Build history of the part. All positions in model axes, mm. A direction names the side the tool comes from. Coordinates: 2 decimals unless noted, no trailing zeros. Order: outer loops, then holes, each group sorted by start corner. A loop starts at its lowest first (then second) coordinate and runs counter-clockwise, first axis right, second up. Notation, with made-up numbers: (48.5, 39.5) - (71.5, 39.5) arc R29 ccw to (71.5, 78.5) - close; hole circle Ø11 at (-30.5, 44). An arc over 180 degrees is marked (long way). Return JSON: item names as keys, results as strings.
from build123d import *

# Parameters (mm, degrees)
SKIZZE1_W                       = 20
SKIZZE1_H                       = 18
SKIZZE1_R                       = 1.5
AUFSATZ_LINEAR_AUSTRAGEN1_DEPTH = 2
SKIZZE2_W                       = 0.8
SKIZZE2_H                       = 0.8
AUFSATZ_LINEAR_AUSTRAGEN2_DEPTH = 8
SKIZZE3_W                       = 1.5
SKIZZE3_H                       = 1.5
AUFSATZ_LINEAR_AUSTRAGEN3_DEPTH = 1.5
LINEARES_MUSTER1_COUNT          = 7
LINEARES_MUSTER1_PITCH          = 2.54


with BuildPart() as part:
    # Skizze1 → Aufsatz-Linear austragen1 (new body)
    with BuildSketch(Plane(origin=(0, 0, 0), x_dir=(1, 0, 0), z_dir=(0, 1, 0))):
        Rectangle(SKIZZE1_W, SKIZZE1_H)
        with Locations((-8, -7)):
            Circle(SKIZZE1_R, mode=Mode.SUBTRACT)
        with Locations((-8, 7)):
            Circle(SKIZZE1_R, mode=Mode.SUBTRACT)
    extrude(amount=AUFSATZ_LINEAR_AUSTRAGEN1_DEPTH)

    # Skizze2 → Aufsatz-Linear austragen2 (add)
    with BuildSketch(Plane.XZ):
        with Locations((8.6, 7.6)):
            Rectangle(SKIZZE2_W, SKIZZE2_H)
    aufsatz_linear_austragen2 = extrude(amount=AUFSATZ_LINEAR_AUSTRAGEN2_DEPTH)

    # Skizze3 → Aufsatz-Linear austragen3 (add)
    with BuildSketch(Plane(origin=(0, 0, 0), x_dir=(-1, 0, 0), z_dir=(0, -1, 0))):
        with Locations((-8.6, -7.6)):
            Rectangle(SKIZZE3_W, SKIZZE3_H)
    aufsatz_linear_austragen3 = extrude(amount=AUFSATZ_LINEAR_AUSTRAGEN3_DEPTH)

    # Lineares Muster1: Aufsatz-Linear austragen2, Aufsatz-Linear austragen3 ×7
    with Locations(*[(0, 0, -i * LINEARES_MUSTER1_PITCH) for i in range(1, LINEARES_MUSTER1_COUNT)]):
        add(aufsatz_linear_austragen2)
        add(aufsatz_linear_austragen3)


solid = part.part
1. Tool access for faces 4 (the flat face through (7.85, -1, 5)), 5 (the flat face through (9, -1, -8.39)), 6 (the flat face through (8.6, -8, 5.1)), 7 (the flat face through (8.6, -4.7, -0.42)), 8 (the flat face through (9, -5, -5)): list every direction of +Z, -Z, +X, -X, +Y, -Y with a clear straight run to the whole face (end or side of a thin tool).
Check values:
{"face 4": "+Z, -Z, -X, -Y", "face 5": "-Z, +X, -X, -Y", "face 6": "+Z, -Z, +X, -X, -Y", "face 7": "+X, -X, -Y", "face 8": "+Z, -Z, +X, -Y"}
2. Cut at A-A on x = -8. Give the cut face in (y, z), plus the area to 3 significant figures.
Check values:
{"outline": "(0, -9) - (2, -9) - (2, -8.5) - (0, -8.5) - close; (0, -5.5) - (2, -5.5) - (2, 5.5) - (0, 5.5) - close; (0, 8.5) - (2, 8.5) - (2, 9) - (0, 9) - close", "area": "24.0 mm²"}
3. Cut at B-B on z = 7.75. Give the cut face in (x, y).
Check values:
{"outline": "(-10, 0) - (-9.3, 0) - (-9.3, 2) - (-10, 2) - close; (-6.7, 0) - (7.85, 0) - (7.85, -1.5) - (8.2, -1.5) - (8.2, -8) - (9, -8) - (9, -1.5) - (9.35, -1.5) - (9.35, 0) - (10, 0) - (10, 2) - (-6.7, 2) - close"}
4. Probe L1, parallel to Z at x = -8, y = 0.7; L2, parallel to X at y = 1.4, z = 7; L3, parallel to Y at x = -8.5, z = 3. List the from-to ranges inside material, lowest first.
Check values:
{"L1": "-9 to -8.5, -5.5 to 5.5, 8.5 to 9", "L2": "-10 to -9.5, -6.5 to 10", "L3": "0 to 2"}
5. Cut at C-C on y = -6.5. Give the cut face in (x, z).
Check values:
{"outline": "(8.2, -8.04) - (9, -8.04) - (9, -7.24) - (8.2, -7.24) - close; (8.2, -5.5) - (9, -5.5) - (9, -4.7) - (8.2, -4.7) - close; (8.2, -2.96) - (9, -2.96) - (9, -2.16) - (8.2, -2.16) - close; (8.2, -0.42) - (9, -0.42) - (9, 0.38) - (8.2, 0.38) - close; (8.2, 2.12) - (9, 2.12) - (9, 2.92) - (8.2, 2.92) - close; (8.2, 4.66) - (9, 4.66) - (9, 5.46) - (8.2, 5.46) - close; (8.2, 7.2) - (9, 7.2) - (9, 8) - (8.2, 8) - close"}
6. Drop flat-ended pins along their axis: pin 1 (4 mm diameter, centred on x = -1, z = -3.5, fed in from -Y); pin 2 (1.2 mm diameter, centred on y = -1, z = -2, fed in from +X); pin 3 (1.6 mm diameter, centred on y = -1, z = 2.5, fed in from -X). Give the stop position or say it passes through.
Check values:
{"pin 1": "y = 0", "pin 2": "x = 9.35", "pin 3": "x = 7.85"}
7. Cut at D-D on z = -6.25. Give the cut face in (x, y), plus the area to 3 significant figures.
Check values:
{"outline": "(-10, 0) - (-9.3, 0) - (-9.3, 2) - (-10, 2) - close; (-6.7, 0) - (10, 0) - (10, 2) - (-6.7, 2) - close", "area": "34.8 mm²"}
8. Mould opens along Z. For faces 1 (the flat face through (9, -4.7, 7.6)), 2 (the flat face through (0, 1, -9)), 3 (the flat face through (8, -1.5, 0)) say: pulls with the +Z half, pulls with the -Z half, needs draft (parallel to the pull), parting line crosses it, or undercut.
Check values:
{"face 1": "needs draft", "face 2": "pulls with the -Z half", "face 3": "undercut"}
